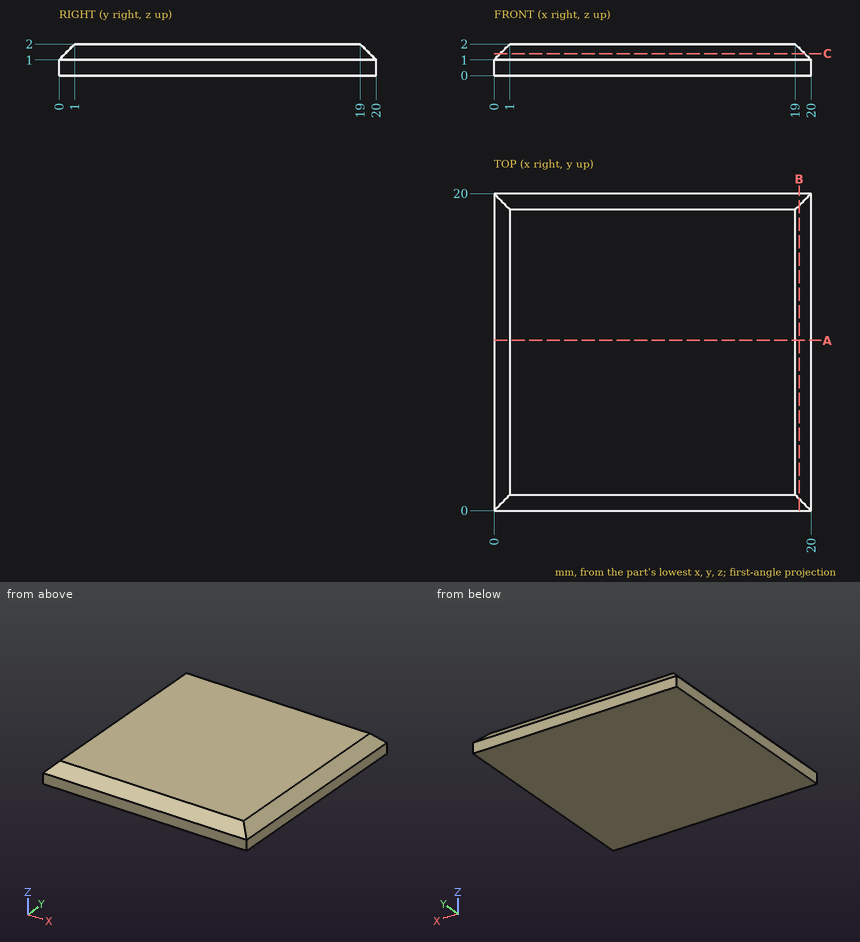
For this review, use the dimensioned drawing (mm, ordinates from the lowest corner) and the shaded views. Round coordinates to 2 decimals unless told otherwise and drop trailing zeros. Loops run counter-clockwise (first coordinate to the right, second up) from the corner with the lowest first, then second, coordinate; pieces in that order, holes last. Notation, with made-up numbers: (-7, 42.25) -> (47, 42.25) arc R18 cw to (47, 46.25) -> close; hole circle Ø11 at (63.25, -18). An arc over 180 degrees is marked (long way). Write item = value, one per line. Start each with the question number.
Item 1: Take a section at B-B on x = 19.25. Give the boundary of the cut face in (y, z).
Item 2: Take a section at A-A on y = 10.75. Give the boundary of the cut face in (x, z).
Item 3: Take a section at C-C on z = 1.4. Give the boundary of the cut face in (x, y).
Item 4: To check wall thickness, follow L1, parallel to X at y = 4, z = 1.4; L2, parallel to Y at x = 18.75, z = 1.6. State the ranges of each line that lie inside material, in increasing order.
Result:
q1.outline = (0, 0) -> (20, 0) -> (20, 1) -> (19.25, 1.75) -> (0.75, 1.75) -> (0, 1) -> close
q2.outline = (0, 0) -> (20, 0) -> (20, 1) -> (19, 2) -> (1, 2) -> (0, 1) -> close
q3.outline = (0.4, 0.4) -> (19.6, 0.4) -> (19.6, 19.6) -> (0.4, 19.6) -> close
q4.L1 = 0.4 to 19.6
q4.L2 = 0.6 to 19.4
